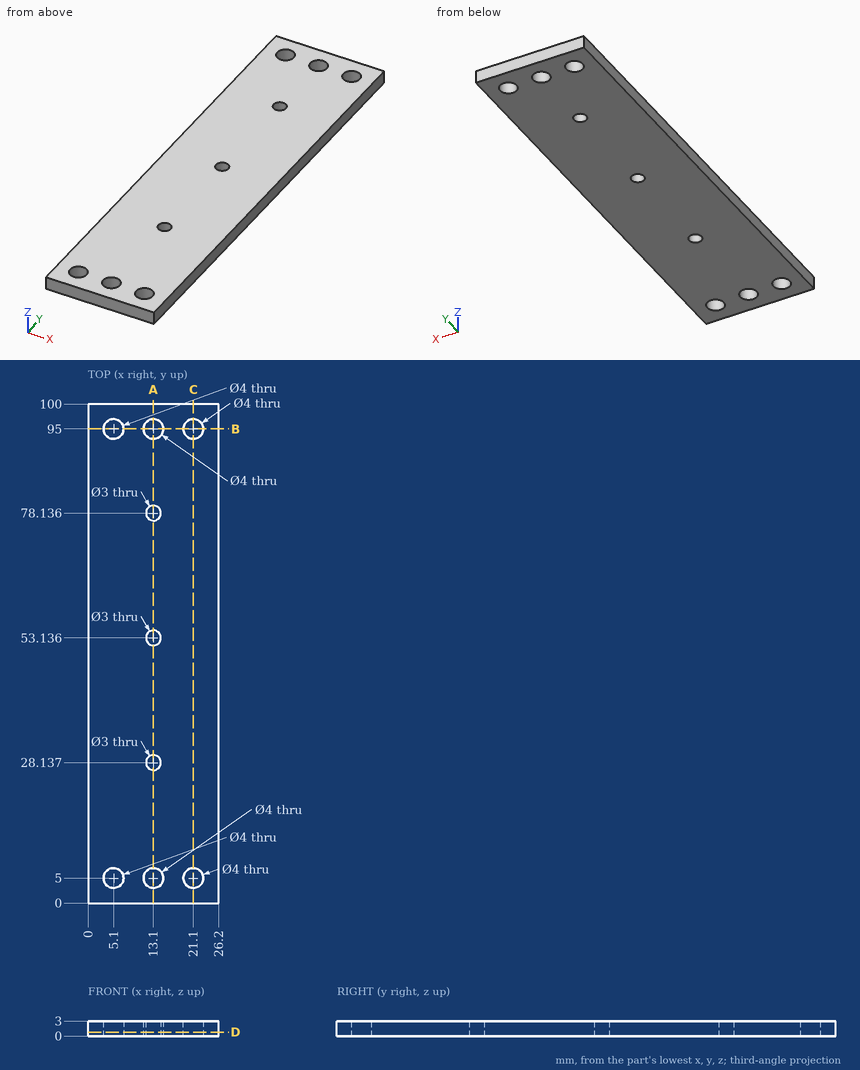
Geometry: see drawing. Coordinates: mm, zero at the bounding-box minimum. Round coordinates to 2 decimals unless told otherwise and drop trailing zeros. Loops run counter-clockwise (first coordinate to the right, second up) from the corner with the lowest first, then second, coordinate; pieces in that order, holes last. Notation, with made-up numbers: (7, -18.75) -> (63, -18.75) arc R29 ccw to (63, 2.25) -> close; hole circle Ø8 at (-22.75, -6.75). An arc over 180 degrees is marked (long way). One line per question, with ' | ' between items. Start each with the question number.
1. Section A-A on x = 13.1. Output: boundary loops of the cut face in (y, z).
2. Section C-C on x = 21.1. Output: boundary loops of the cut face in (y, z).
3. Section B-B on y = 95. Output: boundary loops of the cut face in (x, z).
4. Line query: line 1 along X through (y, z) = (95, 1.5); line 2 along Y through (x, z) = (13.1, 2.3); line 3 along Y through (x, z) = (5.1, 0.85). Output: solid intervals per line, ascending. Write a range as [from, to].
5. Contact query for a flat-ended pin moving along its axis: pin 1 (2.5 mm diameter, centred on x = 13.1, y = 28.14, fed in from -Z). Output: stop coordinate, or through.
6. Section D-D on z = 0.8. Count the separate pieces of the cut face and the enclosed holes in it, and give its area (3 significant figures).
Returned:
1) outline: (0, 0) -> (3, 0) -> (3, 3) -> (0, 3) -> close; (7, 0) -> (26.64, 0) -> (26.64, 3) -> (7, 3) -> close; (29.64, 0) -> (51.64, 0) -> (51.64, 3) -> (29.64, 3) -> close; (54.64, 0) -> (76.64, 0) -> (76.64, 3) -> (54.64, 3) -> close; (79.64, 0) -> (93, 0) -> (93, 3) -> (79.64, 3) -> close; (97, 0) -> (100, 0) -> (100, 3) -> (97, 3) -> close
2) outline: (0, 0) -> (3, 0) -> (3, 3) -> (0, 3) -> close; (7, 0) -> (93, 0) -> (93, 3) -> (7, 3) -> close; (97, 0) -> (100, 0) -> (100, 3) -> (97, 3) -> close
3) outline: (0, 0) -> (3.1, 0) -> (3.1, 3) -> (0, 3) -> close; (7.1, 0) -> (11.1, 0) -> (11.1, 3) -> (7.1, 3) -> close; (15.1, 0) -> (19.1, 0) -> (19.1, 3) -> (15.1, 3) -> close; (23.1, 0) -> (26.2, 0) -> (26.2, 3) -> (23.1, 3) -> close
4) line 1: x = [0, 3.1], [7.1, 11.1], [15.1, 19.1], [23.1, 26.2] | line 2: y = [0, 3], [7, 26.64], [29.64, 51.64], [54.64, 76.64], [79.64, 93], [97, 100] | line 3: y = [0, 3], [7, 93], [97, 100]
5) pin 1: passes through
6) separate pieces: 1 | enclosed holes: 9 | area: 2,520 mm2
